Geometry check sheet. Reference: the model listing, model coordinates, mm. Round coordinates to 2 decimals unless told otherwise and drop trailing zeros. Order: outer loops, then holes, each group sorted by start corner. A loop starts at its lowest first (then second) coordinate and runs counter-clockwise, first axis right, second up.
(1) Cross-section at A-A on y = -114.3. Count the separate pieces of the cut face and the enclosed holes in it, and give its area (3 significant figures).
(2) Thickness scan on L1, parallel to X at y = -127, z = -11.85; L2, parallel to Z at x = 7, y = -10; L3, parallel to Z at x = -24.7, y = -38.1. Record the ranges inside material, lowest first.
(3) Draft check along X on faces 1 (the face through (12.147, -35.608, 11.895)), 2 (the face through (0, 0, -12)), 3 (the face through (-11.328, -27.552, -11.917)). Enter one of: pulls with the +X half, pulls with the -X half, needs draft (parallel to the pull), parting line crosses it, or undercut.
(4) Cross-section at B-B on x = -3.5. Enter the section's corners in (y, z).
(5) Cross-section at C-C on z = -6.5. Enter the section's corners in (x, y).
from build123d import *

# Parameters (mm, degrees)
F0_W     = 50.8
F0_H     = 25.4
F0_W_2   = 47.625
F0_H_2   = 22.225
F1_DEPTH = 152.4
F2_R     = 2.5527
F3_DEPTH = 50.8
F4_R     = 2.5527
F5_DEPTH = 254


# Not quite as in the source:
# - a feature names something its author has since deleted; it is built from what else it names


with BuildPart() as f1:
    # F0 (on Front) → F1 (new body)
    with BuildSketch(Plane.XZ):
        Rectangle(F0_W, F0_H)
        Rectangle(F0_W_2, F0_H_2, mode=Mode.SUBTRACT)
    extrude(amount=F1_DEPTH)

    # F2 (on face) → F3 (cut)
    with BuildSketch(Plane(origin=(-25.4, 0, 0), x_dir=(0, -1, 0), z_dir=(-1, 0, 0))):
        with Locations((139.7, 0)):
            Circle(F2_R)
        with Locations((114.3, 0)):
            Circle(F2_R)
        with Locations((25.4, 0)):
            Circle(F2_R)
        with Locations((101.6, 0)):
            Circle(F2_R)
        with Locations((88.9, 0)):
            Circle(F2_R)
        with Locations((127, 0)):
            Circle(F2_R)
        with Locations((63.5, 0)):
            Circle(F2_R)
        with Locations((76.2, 0)):
            Circle(F2_R)
        with Locations((12.7, 0)):
            Circle(F2_R)
        with Locations((38.1, 0)):
            Circle(F2_R)
        with Locations((50.8, 0)):
            Circle(F2_R)
    extrude(amount=-F3_DEPTH, mode=Mode.SUBTRACT)

    # F4 (on face) → F5 (cut)
    with BuildSketch(Plane(origin=(0, 0, -12.7), x_dir=(1, 0, 0), z_dir=(0, 0, -1))):
        with Locations((12.7, 114.3)):
            Circle(F4_R)
        with Locations((-12.7, 12.7)):
            Circle(F4_R)
        with Locations((12.7, 76.2)):
            Circle(F4_R)
        with Locations((-12.7, 25.4)):
            Circle(F4_R)
        with Locations((12.7, 139.7)):
            Circle(F4_R)
        with Locations((12.7, 50.8)):
            Circle(F4_R)
        with Locations((-12.7, 101.6)):
            Circle(F4_R)
        with Locations((-12.7, 50.8)):
            Circle(F4_R)
        with Locations((12.7, 101.6)):
            Circle(F4_R)
        with Locations((12.7, 12.7)):
            Circle(F4_R)
        with Locations((12.7, 88.9)):
            Circle(F4_R)
        with Locations((-12.7, 127)):
            Circle(F4_R)
        with Locations((12.7, 127)):
            Circle(F4_R)
        with Locations((-12.7, 76.2)):
            Circle(F4_R)
        with Locations((-12.7, 139.7)):
            Circle(F4_R)
        with Locations((-12.7, 88.9)):
            Circle(F4_R)
        with Locations((-12.7, 38.1)):
            Circle(F4_R)
        with Locations((12.7, 38.1)):
            Circle(F4_R)
        with Locations((12.7, 63.5)):
            Circle(F4_R)
        with Locations((-12.7, 114.3)):
            Circle(F4_R)
        with Locations((-12.7, 63.5)):
            Circle(F4_R)
        with Locations((12.7, 25.4)):
            Circle(F4_R)
    extrude(amount=-F5_DEPTH, mode=Mode.SUBTRACT)


solid = f1.part
Found:
1. separate pieces: 6
1. enclosed holes: 0
1. area: 183 mm2
2. L1: x = -25.4 to -15.25, -10.15 to 10.15, 15.25 to 25.4
2. L2: z = -12.7 to -11.11, 11.11 to 12.7
2. L3: z = -12.7 to -2.55, 2.55 to 12.7
3. face 1: undercut
3. face 2: needs draft
3. face 3: undercut
4. outline: (-152.4, -12.7) - (0, -12.7) - (0, -11.11) - (-152.4, -11.11) - close; (-152.4, 11.11) - (0, 11.11) - (0, 12.7) - (-152.4, 12.7) - close
5. outline: (-25.4, -152.4) - (-23.81, -152.4) - (-23.81, 0) - (-25.4, 0) - close; (23.81, -152.4) - (25.4, -152.4) - (25.4, 0) - (23.81, 0) - close
